from build123d import *

# Parameters (mm, degrees)
SKETCH2_R           = 2.65
SKETCH2_R_2         = 2.15
BOSS_EXTRUDE1_DEPTH = 3


with BuildPart() as part:
    # Sketch2 → Boss-Extrude1 (new body)
    with BuildSketch(Plane.XY):
        Polygon((-434.489921235, 165), (-392.489921235, 165), (-392.489921235, 179), (-403.489921235, 190), (-403.489921235, 223), (-423.489921235, 223), (-423.489921235, 190), (-434.489921235, 179), align=None)
        with Locations((-397.489921235, 172)):
            Circle(SKETCH2_R, mode=Mode.SUBTRACT)
        with Locations((-407.489921235, 216)):
            Circle(SKETCH2_R_2, mode=Mode.SUBTRACT)
        with Locations((-407.489921235, 189)):
            Circle(SKETCH2_R_2, mode=Mode.SUBTRACT)
        with Locations((-429.489921235, 172)):
            Circle(SKETCH2_R, mode=Mode.SUBTRACT)
        with Locations((-419.489921235, 189)):
            Circle(SKETCH2_R_2, mode=Mode.SUBTRACT)
        with Locations((-419.489921235, 216)):
            Circle(SKETCH2_R_2, mode=Mode.SUBTRACT)
    extrude(amount=BOSS_EXTRUDE1_DEPTH)


solid = part.part
Geometry check sheet. Reference: the model listing, model coordinates, mm. A direction names the side the tool comes from. Give positions to 0.01 mm unless a question says otherwise; leave off trailing zeros. Order: outer loops, then holes, each group sorted by start corner. A loop starts at its lowest first (then second) coordinate and runs counter-clockwise, first axis right, second up. Notation, with made-up numbers: (53, 82) - (81, 82) arc R32 cw to (81, 117) - close; hole circle Ø1 at (-36, -20). An arc over 180 degrees is marked (long way). Use one line per item in the form item = value.
1) Sectioned sample at D-D (y = 207.5). Record the boundary of the cut face in (x, z).
Working result:
outline = (-423.49, 0) - (-403.49, 0) - (-403.49, 3) - (-423.49, 3) - close
2) Material ranges on probe 1 along X at (y, z) = (172, 2); probe 2 along X at (y, z) = (216, 1.95); probe 3 along Y at (x, z) = (-419, 0.4), recorded low to high. Write a range as from..to.
Working result:
probe_1 = -434.49..-432.14, -426.84..-400.14, -394.84..-392.49
probe_2 = -423.49..-421.64, -417.34..-409.64, -405.34..-403.49
probe_3 = 165..186.91, 191.09..213.91, 218.09..223
3) Sectioned sample at C-C (x = -409). Record the boundary of the cut face in (y, z).
Working result:
outline = (165, 0) - (187.47, 0) - (187.47, 3) - (165, 3) - close; (190.53, 0) - (214.47, 0) - (214.47, 3) - (190.53, 3) - close; (217.53, 0) - (223, 0) - (223, 3) - (217.53, 3) - close
4) Sectioned sample at A-A (y = 216). Record the boundary of the cut face in (x, z), and give its area (3 significant figures).
Working result:
outline = (-423.49, 0) - (-421.64, 0) - (-421.64, 3) - (-423.49, 3) - close; (-417.34, 0) - (-409.64, 0) - (-409.64, 3) - (-417.34, 3) - close; (-405.34, 0) - (-403.49, 0) - (-403.49, 3) - (-405.34, 3) - close
area = 34.2 mm^2
5) Sectioned sample at B-B (z = 0.6). Record the boundary of the cut face in (x, y).
Working result:
outline = (-434.49, 165) - (-392.49, 165) - (-392.49, 179) - (-403.49, 190) - (-403.49, 223) - (-423.49, 223) - (-423.49, 190) - (-434.49, 179) - close; hole circle Ø5.3 at (-429.49, 172); hole circle Ø4.3 at (-419.49, 189); hole circle Ø4.3 at (-419.49, 216); hole circle Ø4.3 at (-407.49, 189); hole circle Ø4.3 at (-407.49, 216); hole circle Ø5.3 at (-397.49, 172)
6) Access from +Z, -Z, +X, -X, +Y, -Y to the whole of each face (thin tool, end or side, straight path). Record for faces 5 (the face through (-403.49, 206, 1)), 6 (the face through (-423.49, 207, 1)), 7 (the face through (-392.49, 172, 1)).
Working result:
face_5 = +Z, -Z, +X, +Y
face_6 = +Z, -Z, -X, +Y
face_7 = +Z, -Z, +X, +Y, -Y
7) Draft check along X on faces 1 (the face through (-405.44, 216.65, 1.48)), 2 (the face through (-434.49, 172, 1)), 3 (the face through (-414, 188, 0)), 4 (the face through (-397.83, 174.63, 1.48)). Enter one of: released by +X, released by -X, zero draft, split by the parting line, or undercut.
Working result:
face_1 = undercut
face_2 = released by -X
face_3 = zero draft
face_4 = undercut
8) Depth check by flat-ended pin: pin 1 Ø1 at (y, z) = (190, 2) entering from +X. Enter the tip coordinate at first touch or a pass-through.
Working result:
pin_1 = -402.99
